The drawing under review shows one solid part. Ordinate dimensions are in mm from its lowest x, y, z. A direction names the side the tool comes from. Round coordinates to 2 decimals unless told otherwise and drop trailing zeros. Loops run counter-clockwise (first coordinate to the right, second up) from the corner with the lowest first, then second, coordinate; pieces in that order, holes last. Notation, with made-up numbers: (3, -2.5) - (13, -2.5) arc R7 ccw to (13, 9.5) - close; hole circle Ø10 at (62.25, 88.25). An arc over 180 degrees is marked (long way). Answer as CSV lines item,"result".
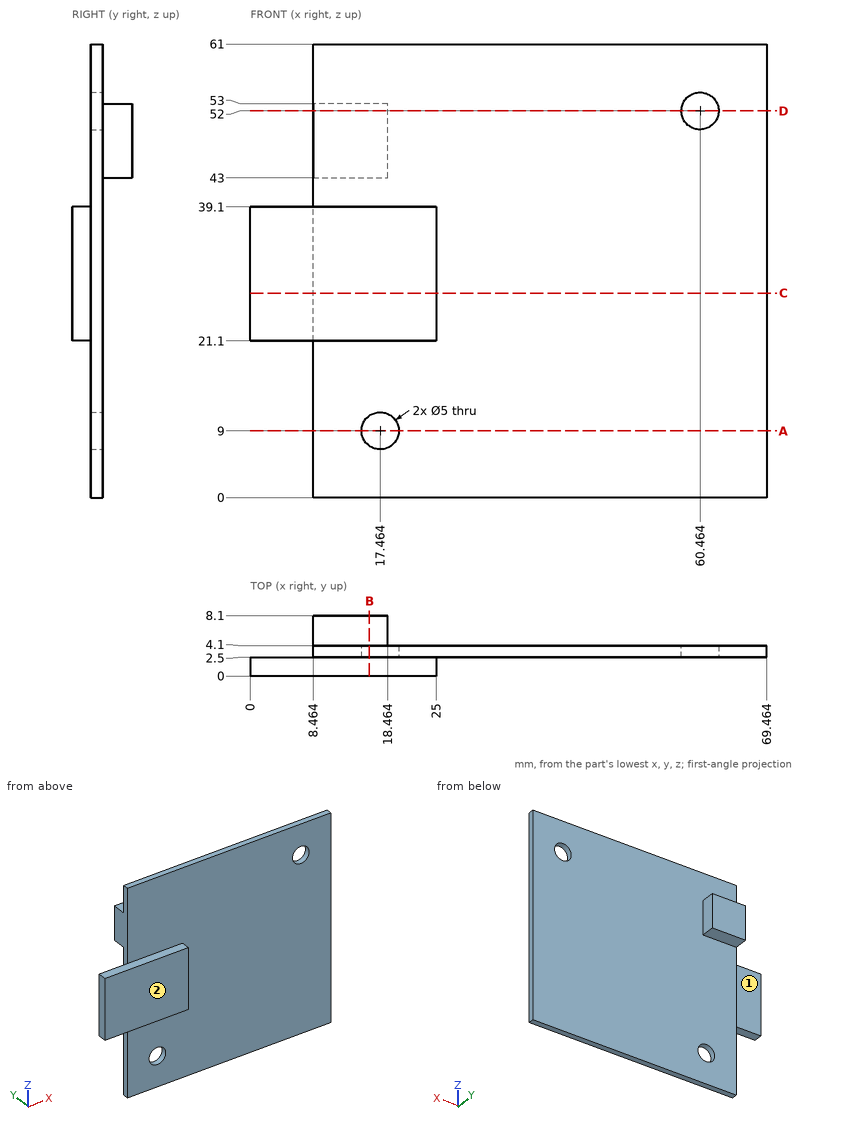
1. Take a section at C-C (z = 27.5). State the section outline as (x, y) points.
Numbers:
outline,"(0, 0) - (25, 0) - (25, 2.5) - (69.46, 2.5) - (69.46, 4.1) - (8.46, 4.1) - (8.46, 2.5) - (0, 2.5) - close"
2. Take a section at A-A (z = 9). State the section outline as (x, y) points, plus the area to 3 significant figures.
Numbers:
outline,"(8.46, 2.5) - (14.96, 2.5) - (14.96, 4.1) - (8.46, 4.1) - close; (19.96, 2.5) - (69.46, 2.5) - (69.46, 4.1) - (19.96, 4.1) - close"
area,"89.6 mm²"
3. Clearance check with flat-ended pins moving along their axes: pin 1 (4 mm diameter, centred on x = 34, z = 33, fed in from +Y); pin 2 (18.5 mm diameter, centred on x = 31, z = 29.5, fed in from -Y); pin 3 (1.2 mm diameter, centred on x = 16, y = 1.5, fed in from -Z); pin 4 (4 mm diameter, centred on x = 35, z = 27.5, fed in from -Y). State where each tip first meets the part, or that it passes through.
Numbers:
pin 1,"stops at y = 4.1"
pin 2,"stops at y = 0"
pin 3,"stops at z = 21.1"
pin 4,"stops at y = 2.5"
4. Take a section at B-B (x = 16). State the section outline as (y, z) points.
Numbers:
outline,"(0, 21.1) - (2.5, 21.1) - (2.5, 11.03) - (4.1, 11.03) - (4.1, 43) - (8.1, 43) - (8.1, 53) - (4.1, 53) - (4.1, 61) - (2.5, 61) - (2.5, 39.1) - (0, 39.1) - close; (2.5, 0) - (4.1, 0) - (4.1, 6.97) - (2.5, 6.97) - close"
5. Take a section at D-D (z = 52). State the section outline as (x, y) points.
Numbers:
outline,"(8.46, 2.5) - (57.96, 2.5) - (57.96, 4.1) - (18.46, 4.1) - (18.46, 8.1) - (8.46, 8.1) - close; (62.96, 2.5) - (69.46, 2.5) - (69.46, 4.1) - (62.96, 4.1) - close"
6. Tool access review of the marked faces 1 and 2: name each direction out of +Z, -Z, +X, -X, +Y, -Y from which nothing blocks a thin tool from reaching the whole face with its end or side.
Numbers:
face 1,"+Z, -Z, -X, +Y"
face 2,"+Z, -Z, +X, -X, -Y"
7. Wall thickness on probe 1 along X at (y, z) = (3.3, 52); probe 2 along Y at (x, z) = (32, 11.5); probe 3 along X at (y, z) = (4, 25): over which ranges is each line inside the solid? List them lowest first.
Numbers:
probe 1,"x = 8.46 to 57.96, 62.96 to 69.46"
probe 2,"y = 2.5 to 4.1"
probe 3,"x = 8.46 to 69.46"
